Source: CAD feature listing. Evaluate the final solid. Frame: model axes, mm. A direction names the side the tool comes from. Give positions to 0.01 mm unless a question says otherwise; leave off trailing zeros. Loops run counter-clockwise (first coordinate to the right, second up) from the corner with the lowest first, then second, coordinate; pieces in that order, holes last. Notation, with made-up numbers: M -12,22 L 3,22 A23 ccw 3,44 Z; hole C 48.5,67.25 d2. An arc over 180 degrees is marked long. Answer in a Markdown table with one row per item.
```python
from build123d import *

# Parameters (mm, degrees)
BOX005_W     = 175
BOX005_H     = 2.5
BOX005_DEPTH = 50
BOX001_W     = 175
BOX001_H     = 47.5
BOX001_DEPTH = 97.5
BOX_W        = 180
BOX_H        = 50
BOX_DEPTH    = 100
BOX002_W     = 2.5
BOX002_H     = 50
BOX002_DEPTH = 87.5
BOX003_W     = 175
BOX003_H     = 2.5
BOX003_DEPTH = 10
BOX004_W     = 175
BOX004_H     = 2.5
BOX004_DEPTH = 5
BOX006_W     = 2.5
BOX006_H     = 50
BOX006_DEPTH = 87.5
BOX007_W     = 2.5
BOX007_H     = 50
BOX007_DEPTH = 87.5


with BuildPart() as back_cutout:
    # Box005 → Box005 (new body)
    with BuildSketch(Plane(origin=(2.5, 47.5, 25), x_dir=(1, 0, 0), z_dir=(0, 0, 1))):
        with Locations((87.5, 1.25)):
            Rectangle(BOX005_W, BOX005_H)
    extrude(amount=BOX005_DEPTH)


with BuildPart() as shell_cutout:
    # Box001 → Box001 (new body)
    with BuildSketch(Plane(origin=(2.5, 0, 2.5), x_dir=(1, 0, 0), z_dir=(0, 0, 1))):
        with Locations((87.5, 23.75)):
            Rectangle(BOX001_W, BOX001_H)
    extrude(amount=BOX001_DEPTH)


with BuildPart() as outer_shell:
    # Box → Box (new body)
    with BuildSketch(Plane.XY):
        with Locations((90, 25)):
            Rectangle(BOX_W, BOX_H)
    extrude(amount=BOX_DEPTH)

    # Cut: cut Shell Cutout
    add(shell_cutout.part, mode=Mode.SUBTRACT)

    # Cut001: cut Back Cutout
    add(back_cutout.part, mode=Mode.SUBTRACT)


with BuildPart() as center_divider:
    # Box002 → Box002 (new body)
    with BuildSketch(Plane(origin=(60, 0, 2.5), x_dir=(1, 0, 0), z_dir=(0, 0, 1))):
        with Locations((1.25, 25)):
            Rectangle(BOX002_W, BOX002_H)
    extrude(amount=BOX002_DEPTH)


with BuildPart() as front_bar:
    # Box003 → Box003 (new body)
    with BuildSketch(Plane(origin=(2.5, 0, 55), x_dir=(1, 0, 0), z_dir=(0, 0, 1))):
        with Locations((87.5, 1.25)):
            Rectangle(BOX003_W, BOX003_H)
    extrude(amount=BOX003_DEPTH)


with BuildPart() as bottom_lip:
    # Box004 → Box004 (new body)
    with BuildSketch(Plane(origin=(2.5, 0, 2.5), x_dir=(1, 0, 0), z_dir=(0, 0, 1))):
        with Locations((87.5, 1.25)):
            Rectangle(BOX004_W, BOX004_H)
    extrude(amount=BOX004_DEPTH)


with BuildPart() as right_divider:
    # Box006 → Box006 (new body)
    with BuildSketch(Plane(origin=(120, 0, 2.5), x_dir=(1, 0, 0), z_dir=(0, 0, 1))):
        with Locations((1.25, 25)):
            Rectangle(BOX006_W, BOX006_H)
    extrude(amount=BOX006_DEPTH)


with BuildPart() as fusion:
    # Box007 → Box007 (new body)
    with BuildSketch(Plane(origin=(60, 0, 2.5), x_dir=(1, 0, 0), z_dir=(0, 0, 1))):
        with Locations((1.25, 25)):
            Rectangle(BOX007_W, BOX007_H)
    extrude(amount=BOX007_DEPTH)

    # Fusion: union Outer Shell, Center Divider, Front Bar, Bottom Lip, Right Divider
    add(outer_shell.part)
    add(center_divider.part)
    add(front_bar.part)
    add(bottom_lip.part)
    add(right_divider.part)


solid = fusion.part
```
1) Pull-direction query (X, two-part tool) for faces 4 (the flat face through (180, 25, 49)), 5 (the flat face through (89, 25, 0)), 6 (the flat face through (150, 25, 2.5)); classes: released by +X, released by -X, zero draft, split by the parting line, or undercut.
Reply:
| item | result |
|---|---|
| face 4 | released by +X |
| face 5 | zero draft |
| face 6 | undercut |
2) Section B-B, the plane z = 44. Return loops of the section in (x, y), then the cut area to 3 significant figures.
Reply:
| item | result |
|---|---|
| outline | M 0,0 L 2.5,0 L 2.5,50 L 0,50 Z; M 60,0 L 62.5,0 L 62.5,50 L 60,50 Z; M 120,0 L 122.5,0 L 122.5,50 L 120,50 Z; M 177.5,0 L 180,0 L 180,50 L 177.5,50 Z |
| area | 500 mm² |
3) Set-up query: faces 1 (the flat face through (150, 2.5, 60)), 2 (the flat face through (90, 0, 57)), 3 (the flat face through (150, 2.5, 5)). Return all of +Z, -Z, +X, -X, +Y, -Y with unobstructed straight access to the full face (end or side cutting, diameter ignored); none if empty.
Reply:
| item | result |
|---|---|
| face 1 | +Z, +Y |
| face 2 | +Z, -Z, +X, -X, -Y |
| face 3 | +Z |
4) Section D-D, the plane z = 86.5. Return loops of the section in (x, y), then the cut area to 3 significant figures.
Reply:
| item | result |
|---|---|
| outline | M 0,0 L 2.5,0 L 2.5,47.5 L 60,47.5 L 60,0 L 62.5,0 L 62.5,47.5 L 120,47.5 L 120,0 L 122.5,0 L 122.5,47.5 L 177.5,47.5 L 177.5,0 L 180,0 L 180,50 L 0,50 Z |
| area | 925 mm² |
5) Pin query (flat end, axial travel): pin 1 Ø1 at (x, y) = (75, 21.5) entering from +Z; pin 2 Ø11 at (x, z) = (89, 58.5) entering from +Y; pin 3 Ø3 at (x, y) = (86, 49) entering from -Z; pin 4 Ø2 at (x, y) = (28, 2) entering from +Z. Return the tip coordinate at first contact, or that it passes through.
Reply:
| item | result |
|---|---|
| pin 1 | stops at z = 2.5 |
| pin 2 | stops at y = 2.5 |
| pin 3 | stops at z = 0 |
| pin 4 | stops at z = 65 |
6) Material intervals for L1, parallel to X at y = 28.5, z = 85.5; L2, parallel to Z at x = 108.5, y = 12.5; L3, parallel to Y at x = 44, z = 17, sorted ascending.
Reply:
| item | result |
|---|---|
| L1 | x = 0 to 2.5, 60 to 62.5, 120 to 122.5, 177.5 to 180 |
| L2 | z = 0 to 2.5 |
| L3 | y = 47.5 to 50 |
7) Section A-A, the plane x = 21. Return loops of the section in (y, z), then the cut area to 3 significant figures.
Reply:
| item | result |
|---|---|
| outline | M 0,0 L 50,0 L 50,25 L 47.5,25 L 47.5,2.5 L 2.5,2.5 L 2.5,7.5 L 0,7.5 Z; M 0,55 L 2.5,55 L 2.5,65 L 0,65 Z; M 47.5,75 L 50,75 L 50,100 L 47.5,100 Z |
| area | 281 mm² |
8) Section C-C, the plane y = 24. Return loops of the section in (x, z), then the cut area to 4 significant figures.
Reply:
| item | result |
|---|---|
| outline | M 0,0 L 180,0 L 180,100 L 177.5,100 L 177.5,2.5 L 122.5,2.5 L 122.5,90 L 120,90 L 120,2.5 L 62.5,2.5 L 62.5,90 L 60,90 L 60,2.5 L 2.5,2.5 L 2.5,100 L 0,100 Z |
| area | 1,375 mm² |
